Part model, mm, in its own coordinate system. Coordinates: 2 decimals unless noted, no trailing zeros. Loops run counter-clockwise (first coordinate to the right, second up) from the corner with the lowest first, then second, coordinate; pieces in that order, holes last. Notation, with made-up numbers: M 40.5,-37 L 57.5,-37 A21 ccw 57.5,-31 Z; hole C 47.5,33.25 d7. An arc over 180 degrees is marked long. Use a Markdown table: item, result. Add a question column.
1) Pull direction Y, two halves, no side cores. Call faces 1 (the flat face through (-24.978, 59.003, 4.93)), 2 (the flat face through (-25.97, 55.52, 4.93)), 3 (the flat face through (-4.643, 27.224, 4.93)): released by +Y, released by -Y, zero draft, split by the parting line, or undercut.
2) Pin check, flat tips, straight feed: pin 1 Ø2 at (x, z) = (-20.5, 3) entering from -Y; pin 2 Ø5 at (y, z) = (49, 6.5) entering from +X; pin 3 Ø4 at (y, z) = (27, 2) entering from -X. Stop position of each tip, or through.
3) Band-saw the part on A-A (x = -16.5). List the corners of the cut face in (y, z).
4) Wall check: probe 1 along X at (y, z) = (25, 5.25); probe 2 along Y at (x, z) = (-31, 2.5); probe 3 along Y at (x, z) = (-29, 2.5). Give the ranges that are in metal, low to high. Write a range as from..to.
from build123d import *

# Parameters (mm, degrees)
SKETCH1_R           = 2.75
BOSS_EXTRUDE1_DEPTH = 10


with BuildPart() as part:
    # Sketch1 → Boss-Extrude1 (new body)
    with BuildSketch(Plane.XY):
        with BuildLine():
            Line((-5.771263161, 52.493232874), (2.09039449, 5.62407778))
            ThreePointArc((2.09039449, 5.62407778), (2.348768815, 5.521167001), (2.602096685, 5.4063937))
            Line((2.602096685, 5.4063937), (2.367387425, 4.404029607))
            ThreePointArc((2.367387425, 4.404029607), (2.707371965, 4.203586212), (3.030487733, 3.976951609))
            Line((3.030487733, 3.976951609), (3.922838506, 4.539971151))
            ThreePointArc((3.922838506, 4.539971151), (4.206602502, 4.278375322), (4.472961167, 3.999077193))
            Line((4.472961167, 3.999077193), (3.872529953, 3.162832869))
            ThreePointArc((3.872529953, 3.162832869), (4.109928346, 2.847540868), (4.321719082, 2.514506746))
            Line((4.321719082, 2.514506746), (5.361601948, 2.693181121))
            ThreePointArc((5.361601948, 2.693181121), (5.523657306, 2.342906308), (5.662857859, 1.982937436))
            Line((5.662857859, 1.982937436), (4.788114901, 1.440123498))
            ThreePointArc((4.788114901, 1.440123498), (4.886785392, 1.05798324), (4.955007877, 0.669251025))
            Line((4.955007877, 0.669251025), (5.984110097, 0.436378678))
            ThreePointArc((5.984110097, 0.436378678), (5.999785357, 0.050751048), (5.990635775, -0.335086571))
            Line((5.990635775, -0.335086571), (4.97475276, -0.501831621))
            ThreePointArc((4.97475276, -0.501831621), (4.919673661, -0.892642746), (4.833941641, -1.277892098))
            Line((4.833941641, -1.277892098), (5.695591729, -1.886858462))
            ThreePointArc((5.695591729, -1.886858462), (5.562500476, -2.2491306), (5.4063937, -2.602096685))
            Line((5.4063937, -2.602096685), (4.404029607, -2.367387425))
            ThreePointArc((4.404029607, -2.367387425), (4.203586212, -2.707371965), (3.976951609, -3.030487733))
            Line((3.976951609, -3.030487733), (4.539971151, -3.922838506))
            ThreePointArc((4.539971151, -3.922838506), (4.278375322, -4.206602502), (3.999077193, -4.472961167))
            Line((3.999077193, -4.472961167), (3.162832869, -3.872529953))
            ThreePointArc((3.162832869, -3.872529953), (2.847540868, -4.109928346), (2.514506746, -4.321719082))
            Line((2.514506746, -4.321719082), (2.693181121, -5.361601948))
            ThreePointArc((2.693181121, -5.361601948), (2.342906308, -5.523657306), (1.982937436, -5.662857859))
            Line((1.982937436, -5.662857859), (1.440123498, -4.788114901))
            ThreePointArc((1.440123498, -4.788114901), (1.05798324, -4.886785392), (0.669251025, -4.955007877))
            Line((0.669251025, -4.955007877), (0.436378678, -5.984110097))
            ThreePointArc((0.436378678, -5.984110097), (0.050751048, -5.999785357), (-0.335086571, -5.990635775))
            Line((-0.335086571, -5.990635775), (-0.501831621, -4.97475276))
            ThreePointArc((-0.501831621, -4.97475276), (-0.892642746, -4.919673661), (-1.277892098, -4.833941641))
            Line((-1.277892098, -4.833941641), (-1.886858462, -5.695591729))
            ThreePointArc((-1.886858462, -5.695591729), (-2.2491306, -5.562500476), (-2.602096685, -5.4063937))
            Line((-2.602096685, -5.4063937), (-2.367387425, -4.404029607))
            ThreePointArc((-2.367387425, -4.404029607), (-2.707371965, -4.203586212), (-3.030487733, -3.976951609))
            Line((-3.030487733, -3.976951609), (-3.922838506, -4.539971151))
            ThreePointArc((-3.922838506, -4.539971151), (-4.206602502, -4.278375322), (-4.472961167, -3.999077193))
            Line((-4.472961167, -3.999077193), (-3.872529953, -3.162832869))
            ThreePointArc((-3.872529953, -3.162832869), (-4.109928346, -2.847540868), (-4.321719082, -2.514506746))
            Line((-4.321719082, -2.514506746), (-5.361601948, -2.693181121))
            ThreePointArc((-5.361601948, -2.693181121), (-5.523657306, -2.342906308), (-5.662857859, -1.982937436))
            Line((-5.662857859, -1.982937436), (-4.788114901, -1.440123498))
            ThreePointArc((-4.788114901, -1.440123498), (-4.886785392, -1.05798324), (-4.955007877, -0.669251025))
            Line((-4.955007877, -0.669251025), (-5.984110097, -0.436378678))
            ThreePointArc((-5.984110097, -0.436378678), (-5.999785357, -0.050751048), (-5.990635775, 0.335086571))
            Line((-5.990635775, 0.335086571), (-4.97475276, 0.501831621))
            ThreePointArc((-4.97475276, 0.501831621), (-4.919673661, 0.892642746), (-4.833941641, 1.277892098))
            Line((-4.833941641, 1.277892098), (-5.695591729, 1.886858462))
            ThreePointArc((-5.695591729, 1.886858462), (-5.562500476, 2.2491306), (-5.4063937, 2.602096685))
            Line((-5.4063937, 2.602096685), (-4.404029607, 2.367387425))
            ThreePointArc((-4.404029607, 2.367387425), (-4.203586212, 2.707371965), (-3.976951609, 3.030487733))
            Line((-3.976951609, 3.030487733), (-4.539971151, 3.922838506))
            ThreePointArc((-4.539971151, 3.922838506), (-4.278375322, 4.206602502), (-3.999077193, 4.472961167))
            Line((-3.999077193, 4.472961167), (-3.162832869, 3.872529953))
            ThreePointArc((-3.162832869, 3.872529953), (-2.847540868, 4.109928346), (-2.514506746, 4.321719082))
            Line((-2.514506746, 4.321719082), (-2.693181121, 5.361601948))
            ThreePointArc((-2.693181121, 5.361601948), (-2.342906308, 5.523657306), (-1.982937436, 5.662857859))
            Line((-1.982937436, 5.662857859), (-1.630850624, 5.095471066))
            Line((-1.630850624, 5.095471066), (-1.721009902, 5.747880037))
            Line((-1.721009902, 5.747880037), (-7.647759844, 49.309063447))
            Line((-7.647759844, 49.309063447), (-44.816075509, 61.905592465))
            Line((-44.816075509, 61.905592465), (-43.65479695, 65.33215291))
            Line((-43.65479695, 65.33215291), (-5.771263161, 52.493232874))
        make_face()
        Circle(SKETCH1_R, mode=Mode.SUBTRACT)
    extrude(amount=BOSS_EXTRUDE1_DEPTH)


solid = part.part
Entries:
| question | item | result |
|---|---|---|
| 1 | face 1 | released by +Y |
| 1 | face 2 | released by -Y |
| 1 | face 3 | undercut |
| 2 | pin 1 | y = 53.33 |
| 2 | pin 2 | x = -4.77 |
| 2 | pin 3 | x = -4.88 |
| 3 | outline | M 52.31,0 L 56.13,0 L 56.13,10 L 52.31,10 Z |
| 4 | probe 1 | -4.34..-1.16 |
| 4 | probe 2 | 57.22..61.04 |
| 4 | probe 3 | 56.55..60.37 |
